Part print with two shaded views. Sizes in mm from the minimum x, y, z corner. A direction names the side the tool comes from. Coordinates: 2 decimals unless noted, no trailing zeros. Order: outer loops, then holes, each group sorted by start corner. A loop starts at its lowest first (then second) coordinate and runs counter-clockwise, first axis right, second up. Notation, with made-up numbers: (66.5, 45) - (84.5, 45) arc R11 ccw to (84.5, 63) - close; hole circle Ø4 at (-31.5, -25). An arc over 180 degrees is marked (long way). Return JSON: item names as keys, results as strings.
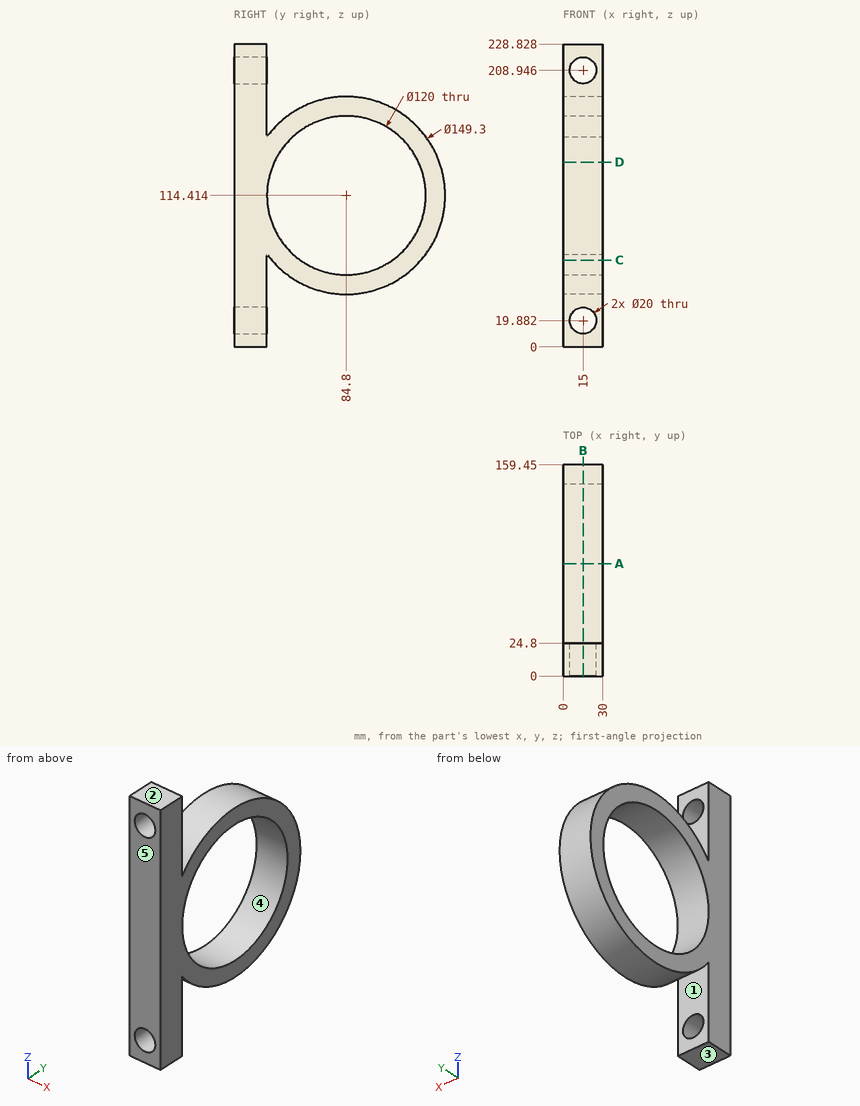
Item 1: Which spindle directions (+Z, -Z, +X, -X, +Y, -Y) get a long thin tool onto all of the face, cutting with end or side? Do the marked faces 1 and 2. Say none if no direction does.
Findings below:
{"face 1": "-Z, +X, -X", "face 2": "+Z, +X, -X, +Y, -Y"}
Item 2: Band-saw the part on B-B, the plane x = 15. Count the separate pieces of the cut face and the enclosed holes in it.
Findings below:
{"separate pieces": "3", "enclosed holes": "1"}
Item 3: Band-saw the part on D-D, the plane z = 139.5. List the corners of the cut face in (x, y) (1 decimal), then the cut area to 3 significant figures.
Findings below:
{"outline": "(0, 0) - (30, 0) - (30, 30.3) - (0, 30.3) - close; (0, 139.3) - (30, 139.3) - (30, 155.1) - (0, 155.1) - close", "area": "1,380 mm²"}
Item 4: Band-saw the part on A-A, the plane y = 84.8. List the corners of the cut face in (x, z) (1 decimal).
Findings below:
{"outline": "(0, 39.8) - (30, 39.8) - (30, 54.4) - (0, 54.4) - close; (0, 174.4) - (30, 174.4) - (30, 189.1) - (0, 189.1) - close"}
Item 5: Mould opens along Y. For the marked faces 3, 4 and 5 say: released by +Y, released by -Y, zero draft, split by the parting line, or undercut.
Findings below:
{"face 3": "zero draft", "face 4": "undercut", "face 5": "released by -Y"}
Item 6: Band-saw the part on C-C, the plane z = 65.5. List the corners of the cut face in (x, y), then the cut area to 3 significant figures.
Findings below:
{"outline": "(0, 0) - (30, 0) - (30, 24.8) - (0, 24.8) - close; (0, 28.41) - (30, 28.41) - (30, 50.05) - (0, 50.05) - close; (0, 119.55) - (30, 119.55) - (30, 141.19) - (0, 141.19) - close", "area": "2,040 mm²"}
Item 7: Wall check: L1, parallel to Y at x = 23.25, z = 167 (1 decimal); L2, parallel to Z at x = 1.5, y = 86 (1 decimal); L3, parallel to Y at x = 24.75, z = 31. Give the ranges that are in metal, low to high. Write a range as [from, to].
Findings below:
{"L1": "y = [0, 24.8], [31.8, 55.9], [113.7, 137.8]", "L2": "z = [39.8, 54.4], [174.4, 189.1]", "L3": "y = [0, 24.8]"}
Item 8: Drop flat-ended pins along their axis: P1, Ø12, axis at x = 16, y = 56.5, coming from the +Z side (1 decimal); P2, Ø10, axis at x = 22, y = 37.5, coming from the -Z side (1 decimal); P3, Ø16, axis at x = 15, z = 19.88, coming from the -Y side; P4, Ø15, axis at x = 15, z = 32, coming from the +Y side. Give the stop position or say it passes through.
Findings below:
{"P1": "stops at z = 185.7", "P2": "stops at z = 52.9", "P3": "passes through", "P4": "stops at y = 24.8"}
